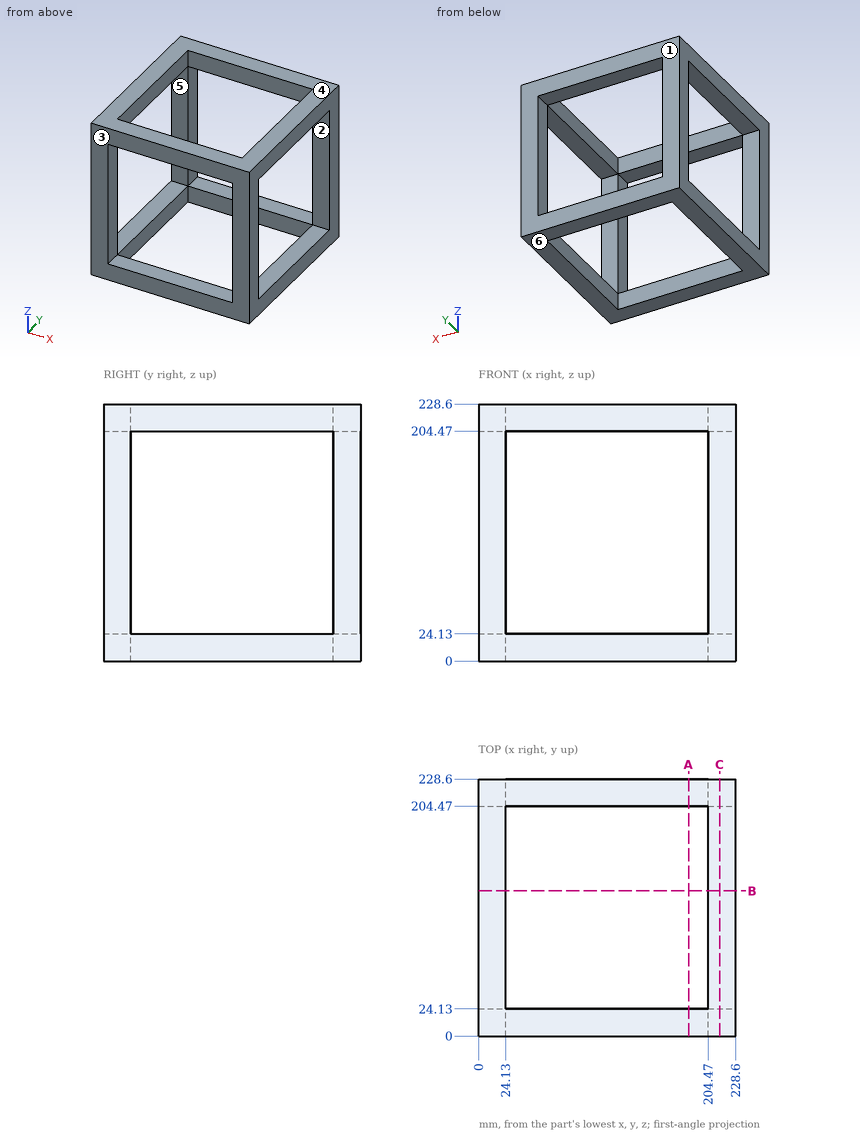
Geometry check sheet. Reference: drawing and pictorial views, mm from the part's lowest x, y, z. A direction names the side the tool comes from. Round coordinates to 2 decimals unless told otherwise and drop trailing zeros. Loops run counter-clockwise (first coordinate to the right, second up) from the corner with the lowest first, then second, coordinate; pieces in that order, holes last. Notation, with made-up numbers: (60, -17) - (69, -17) arc R23 ccw to (69, 5) - close; hole circle Ø11 at (7.5, -32.75). An arc over 180 degrees is marked (long way). Answer in a Markdown table with one row per item. Add a question column.
Q1. Section check C-C on x = 214.5. Enter the section's corners in (y, z).
Q2. Gauge pin test, flat ends, axial feed: pin 1 (12 mm diameter, centred on y = 215.5, z = 129, fed in from -X); pin 2 (5 mm diameter, centred on x = 133.5, y = 200.5, fed in from -Z). Record the tip position at first contact, or that the pin passes through.
Q3. Section check A-A on x = 187. Enter the section's corners in (y, z).
Q4. Release check for a two-part mould opening along Y. For the marked faces 1, 2, 3 and 4 record: pulls with the +Y half, pulls with the -Y half, needs draft (parallel to the pull), parting line crosses it, or undercut.
Q5. Material ranges on line 1 (Y direction, x = 206.5, z = 99.5), recorded low to high.
Q6. Tool access check on the marked faces 5 and 6. Record the directions out of +Z, -Z, +X, -X, +Y, -Y that give a thin tool (end or side, any length) a straight path to the whole face; none if there is none.
Found:
| question | item | result |
|---|---|---|
| 1 | outline | (0, 0) - (228.6, 0) - (228.6, 228.6) - (0, 228.6) - close; hole (24.13, 24.13) - (204.47, 24.13) - (204.47, 204.47) - (24.13, 204.47) - close |
| 2 | pin 1 | stops at x = 0 |
| 2 | pin 2 | passes through |
| 3 | outline | (0, 0) - (24.13, 0) - (24.13, 24.13) - (0, 24.13) - close; (0, 204.47) - (24.13, 204.47) - (24.13, 228.6) - (0, 228.6) - close; (204.47, 0) - (228.6, 0) - (228.6, 24.13) - (204.47, 24.13) - close; (204.47, 204.47) - (228.6, 204.47) - (228.6, 228.6) - (204.47, 228.6) - close |
| 4 | face 1 | pulls with the +Y half |
| 4 | face 2 | undercut |
| 4 | face 3 | pulls with the -Y half |
| 4 | face 4 | needs draft |
| 5 | line 1 | y = 0 to 24.13, 204.47 to 228.6 |
| 6 | face 5 | +X, -X |
| 6 | face 6 | -Z, +X, -X, +Y, -Y |
